from build123d import *
from OCP.BRepFilletAPI import BRepFilletAPI_MakeFillet

# Parameters (mm, degrees)
SKETCH1_W           = 8
SKETCH1_H           = 15
BOSS_EXTRUDE1_DEPTH = 22
CUT_EXTRUDE1_START  = 18.5
SKETCH2_R           = 1.4
CUT_EXTRUDE1_DEPTH  = 10
SKETCH3_W           = 8
SKETCH3_H           = 15
BOSS_EXTRUDE2_DEPTH = 6
BOSS_EXTRUDE3_START = -6
BOSS_EXTRUDE3_DEPTH = 5
BOSS_EXTRUDE4_START = -11
SKETCH5_W           = 34.3
SKETCH5_H           = 15
BOSS_EXTRUDE4_DEPTH = 5
SKETCH7_R           = 2.55
SKETCH7_R_2         = 2.4
CUT_EXTRUDE2_DEPTH  = 48.05677422
FILLET1_R           = 5
FILLET1_R_2         = 2


with BuildPart() as part:
    # Sketch1 → Boss-Extrude1 (new body)
    with BuildSketch(Plane.XY):
        with Locations((0, 11)):
            Rectangle(SKETCH1_W, SKETCH1_H)
    extrude(amount=BOSS_EXTRUDE1_DEPTH)

    # Sketch2 → Cut-Extrude1 (cut)
    with BuildSketch(Plane(origin=(0, 0, 0), x_dir=(1, 0, 0), z_dir=(0, 1, 0)).offset(CUT_EXTRUDE1_START)):
        with Locations(Location((0, -7, 0), (0, 0, 90))):
            Circle(SKETCH2_R)
        with Locations(Location((0, -17, 0), (0, 0, 90))):
            Circle(SKETCH2_R)
    extrude(amount=-CUT_EXTRUDE1_DEPTH, mode=Mode.SUBTRACT)

    # Sketch3 → Boss-Extrude2 (add)
    with BuildSketch(Plane.XY):
        with Locations((0, 11)):
            Rectangle(SKETCH3_W, SKETCH3_H)
    extrude(amount=-BOSS_EXTRUDE2_DEPTH)

    # Sketch4 → Boss-Extrude3 (add)
    with BuildSketch(Plane.XY.offset(BOSS_EXTRUDE3_START)):
        Polygon((-16, -13.5), (4, -13.5), (4, 13.5), (-30.3, 13.5), (-30.3, 5.25), (-18.3, 5.25), (-18.3, -6.75), (-30.3, -6.75), (-30.3, -13.5), align=None)
    extrude(amount=-BOSS_EXTRUDE3_DEPTH)

    # Sketch5 → Boss-Extrude4 (add)
    with BuildSketch(Plane.XY.offset(BOSS_EXTRUDE4_START)):
        with Locations((-13.15, 21)):
            Rectangle(SKETCH5_W, SKETCH5_H)
    extrude(amount=BOSS_EXTRUDE4_DEPTH)

    # Sketch7 → Cut-Extrude2 (cut, through all)
    with BuildSketch(Plane.XY):
        with Locations((-25.3, 19.25)):
            Circle(SKETCH7_R)
        with Locations((-25.3, 9.25)):
            Circle(SKETCH7_R_2)
    extrude(amount=-CUT_EXTRUDE2_DEPTH, mode=Mode.SUBTRACT)

    # Fillet1
    fillet1_edges_1 = [part.edges().sort_by_distance(p)[0] for p in [
        (-4, 11, -6),
        (0, 18.5, -6),
        (-18.3, -6.75, -8.5),
        (-18.3, 5.25, -8.5),
        (-30.3, 5.25, -8.5),
        (4, -13.5, -8.5),
        (4, 11, 22),
        (4, 28.5, -8.5),
        (-30.3, 28.5, -8.5),
        (4, 3.5, 8),
    ]]
    fillet1_edges_2 = [part.edges().sort_by_distance(p)[0] for p in [
        (-30.3, -6.75, -8.5),
        (-30.3, -13.5, -8.5),
    ]]
    fillet1 = BRepFilletAPI_MakeFillet(part.part.solid().wrapped)
    for e in fillet1_edges_1:
        fillet1.Add(FILLET1_R - 0.0001, e.wrapped)
    for e in fillet1_edges_2:
        fillet1.Add(FILLET1_R_2 - 0.0001, e.wrapped)
    add(Compound.cast(fillet1.Shape()), mode=Mode.REPLACE)  # a hair under: the kernel refuses the full size


solid = part.part
Geometry check sheet. Reference: the model listing, model coordinates, mm. A direction names the side the tool comes from. Give positions to 0.01 mm unless a question says otherwise; leave off trailing zeros. Order: outer loops, then holes, each group sorted by start corner. A loop starts at its lowest first (then second) coordinate and runs counter-clockwise, first axis right, second up. Notation, with made-up numbers: (74, -3.5) - (81, -3.5) arc R18 ccw to (81, 30.5) - close; hole circle Ø6 at (-20, 23.5). An arc over 180 degrees is marked (long way). Answer as a JSON object with one key per item and string values.
(1) Cross-section at B-B (x = -22). Record the cut outline in (y, z), then the cut area to 3 significant figures.
Report:
{"outline": "(-13.5, -11) - (-6.58, -11) - (-6.58, -6) - (-13.5, -6) - close; (5.08, -11) - (28.5, -11) - (28.5, -6) - (5.08, -6) - close", "area": "152 mm^2"}
(2) Depth check by flat-ended pin: pin 1 Ø0.6 at (y, z) = (-1, -8) entering from -X; pin 2 Ø8 at (x, y) = (-15, 9.5) entering from +Z; pin 3 Ø16.5 at (y, z) = (10, 8) entering from -X. Enter the tip coordinate at first touch or a pass-through.
Report:
{"pin 1": "x = -18.3", "pin 2": "z = -6", "pin 3": "x = -4"}
(3) Tool access check on faces 5 (the flat face through (0, 8.5, 7)), 6 (the flat face through (-26, -6.75, -8)), 7 (the flat face through (0, 18.5, 11)). Record the directions out of +Z, -Z, +X, -X, +Y, -Y that give a thin tool (end or side, any length) a straight path to the whole face; none if there is none.
Report:
{"face 5": "+Y", "face 6": "+Z, -Z, -X", "face 7": "+Z, +X, -X, +Y"}
(4) Draft check along X on faces 1 (the flat face through (-18.3, -1, -8)), 2 (the cylindrical face through (-27.07, 10.87, -8.46)), 3 (the cylindrical face through (2.5, 27.07, -8.46)), 4 (the flat face through (-15, -13.5, -8)). Enter one of: released by +X, released by -X, zero draft, split by the parting line, or undercut.
Report:
{"face 1": "released by -X", "face 2": "undercut", "face 3": "released by +X", "face 4": "zero draft"}
(5) Cross-section at A-A (z = 7). Record the cut outline in (x, y), then the cut area to 3 significant figures.
Report:
{"outline": "(-4, 3.5) - (-1, 3.5) arc R5 ccw to (4, 8.5) - (4, 18.5) - (1.4, 18.5) - (1.4, 8.5) - (-1.4, 8.5) - (-1.4, 18.5) - (-4, 18.5) - close", "area": "86.6 mm^2"}
(6) Cross-section at D-D (x = -5.5). Record the cut outline in (y, z), then the cut area to 3 significant figures.
Report:
{"outline": "(-13.5, -11) - (28.5, -11) - (28.5, -6) - (23.5, -6) arc R5 cw to (20, -4.57) - (3.5, -4.57) - (3.5, -6) - (-13.5, -6) - close", "area": "235 mm^2"}
(7) Material ranges on line 1 (X direction, y = 14, z = 7); line 2 (X direction, y = 19, z = -7); line 3 (X direction, y = 11, z = 15.5), recorded low to high.
Report:
{"line 1": "-4 to -1.4, 1.4 to 4", "line 2": "-30.3 to -27.84, -22.76 to 4", "line 3": "-4 to 4"}
(8) Cross-section at C-C (y = 19.25). Record the cut outline in (x, z), then the cut area to 3 significant figures.
Report:
{"outline": "(-30.3, -11) - (-27.85, -11) - (-27.85, -6) - (-30.3, -6) - close; (-22.75, -11) - (4, -11) - (4, -3.63) - (-4.75, -3.63) arc R5 cw to (-9, -6) - (-22.75, -6) - close", "area": "170 mm^2"}
